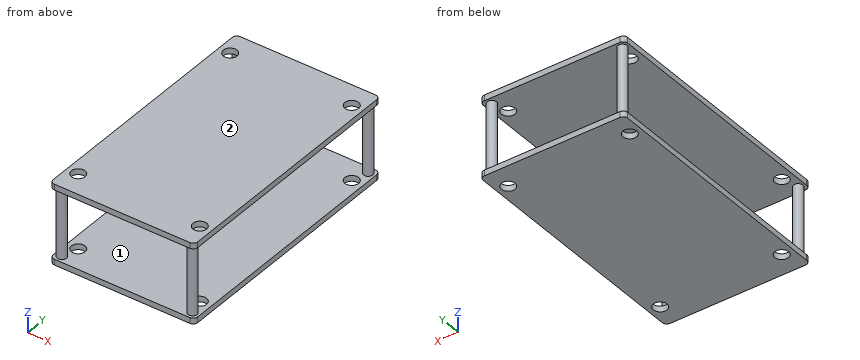
```python
from build123d import *

# Parameters (mm, degrees)
SKETCH1_W           = 63
SKETCH1_H           = 110
SKETCH1_R           = 3
BOSS_EXTRUDE1_DEPTH = 2.5
SKETCH3_R           = 2
BOSS_EXTRUDE3_DEPTH = 30
FILLET2_R           = 2
FILLET3_R           = 2
FILLET4_R           = 2
FILLET5_R           = 2
SKETCH5_W           = 63
SKETCH5_H           = 110
SKETCH5_R           = 3
BOSS_EXTRUDE5_DEPTH = 2.5
FILLET10_R          = 2
FILLET11_R          = 2
FILLET12_R          = 2
FILLET13_R          = 2


with BuildPart() as part:
    # Sketch1 → Boss-Extrude1 (new body)
    with BuildSketch(Plane.XY):
        Rectangle(SKETCH1_W, SKETCH1_H)
        with Locations((-26.5, 45)):
            Circle(SKETCH1_R, mode=Mode.SUBTRACT)
        with Locations((-26.5, -45)):
            Circle(SKETCH1_R, mode=Mode.SUBTRACT)
        with Locations((26.5, -45)):
            Circle(SKETCH1_R, mode=Mode.SUBTRACT)
        with Locations((26.5, 45)):
            Circle(SKETCH1_R, mode=Mode.SUBTRACT)
    extrude(amount=BOSS_EXTRUDE1_DEPTH)

    # Sketch3 → Boss-Extrude3 (add)
    with BuildSketch(Plane.XY.offset(2.5)):
        with Locations(Location((-28.5, 52, 0), (0, 0, 180))):
            Circle(SKETCH3_R)
        with Locations(Location((28.5, 52, 0), (0, 0, 180))):
            Circle(SKETCH3_R)
        with Locations(Location((28.5, -52, 0), (0, 0, 180))):
            Circle(SKETCH3_R)
        with Locations(Location((-28.5, -52, 0), (0, 0, 180))):
            Circle(SKETCH3_R)
    extrude(amount=BOSS_EXTRUDE3_DEPTH)

    # Fillet2
    fillet2_edges = [part.edges().sort_by_distance(p)[0] for p in [
        (31.5, -55, 1.25),
    ]]
    fillet(fillet2_edges, radius=FILLET2_R)

    # Fillet3
    fillet3_edges = [part.edges().sort_by_distance(p)[0] for p in [
        (31.5, 55, 1.25),
    ]]
    fillet(fillet3_edges, radius=FILLET3_R)

    # Fillet4
    fillet4_edges = [part.edges().sort_by_distance(p)[0] for p in [
        (-31.5, 55, 1.25),
    ]]
    fillet(fillet4_edges, radius=FILLET4_R)

    # Fillet5
    fillet5_edges = [part.edges().sort_by_distance(p)[0] for p in [
        (-31.5, -55, 1.25),
    ]]
    fillet(fillet5_edges, radius=FILLET5_R)

    # Sketch5 → Boss-Extrude5 (add)
    with BuildSketch(Plane.XY.offset(32.5)):
        Rectangle(SKETCH5_W, SKETCH5_H)
        with Locations((-26.5, 45)):
            Circle(SKETCH5_R, mode=Mode.SUBTRACT)
        with Locations((-26.5, -45)):
            Circle(SKETCH5_R, mode=Mode.SUBTRACT)
        with Locations((26.5, -45)):
            Circle(SKETCH5_R, mode=Mode.SUBTRACT)
        with Locations((26.5, 45)):
            Circle(SKETCH5_R, mode=Mode.SUBTRACT)
    extrude(amount=BOSS_EXTRUDE5_DEPTH)

    # Fillet10
    fillet10_edges = [part.edges().sort_by_distance(p)[0] for p in [
        (31.5, 55, 33.75),
    ]]
    fillet(fillet10_edges, radius=FILLET10_R)

    # Fillet11
    fillet11_edges = [part.edges().sort_by_distance(p)[0] for p in [
        (31.5, -55, 33.75),
    ]]
    fillet(fillet11_edges, radius=FILLET11_R)

    # Fillet12
    fillet12_edges = [part.edges().sort_by_distance(p)[0] for p in [
        (-31.5, -55, 33.75),
    ]]
    fillet(fillet12_edges, radius=FILLET12_R)

    # Fillet13
    fillet13_edges = [part.edges().sort_by_distance(p)[0] for p in [
        (-31.5, 55, 33.75),
    ]]
    fillet(fillet13_edges, radius=FILLET13_R)


solid = part.part
```
Verification items for the finished model (mm, model axes). Face numbers are marked on the shaded views. Coordinates: 2 decimals unless noted, no trailing zeros. Write each loop counter-clockwise with the first axis right and the second up, starting at its lowest first coordinate (ties: lowest second). Pieces come first, ordered by that corner, then holes. Notation, with made-up numbers: M 72.5,45 L 104.5,45 A9 cw 104.5,59 Z; hole C 38.25,88.25 d2. An arc over 180 degrees is marked long. Answer as a JSON object with one key per item and string values. Group by question number.
(1) Cross-section at D-D, the plane y = 22.5. Record the cut outline in (x, z), and give its area (3 significant figures).
(2) Cross-section at B-B, the plane x = -12. Record the cut outline in (y, z), and give its area (3 significant figures).
(3) Cross-section at A-A, the plane y = -45. Record the cut outline in (x, z), and give its area (3 significant figures).
(4) Material ranges on line 1 (Y direction, x = -26.5, z = 33.5); line 2 (Z direction, x = 20, y = 38), recorded low to high.
(5) Release check for a two-part mould opening along Y. For the marked faces 1 and 2 record: +Y half, -Y half, draft (parallel to the pull), parting line (faces both ways), or undercut.
(6) Cross-section at C-C, the plane z = 25. Record the cut outline in (x, y).
(7) Gauge pin test, flat end, axial feed: pin 1 (3.5 mm diameter, centred on x = -26.5, y = -45, fed in from +Z). Record the tip position at first contact, or that the pin passes through.
Reply:
{
 "1": {"outline": "M -31.5,0 L 31.5,0 L 31.5,2.5 L -31.5,2.5 Z; M -31.5,32.5 L 31.5,32.5 L 31.5,35 L -31.5,35 Z", "area": "315 mm²"},
 "2": {"outline": "M -55,0 L 55,0 L 55,2.5 L -55,2.5 Z; M -55,32.5 L 55,32.5 L 55,35 L -55,35 Z", "area": "550 mm²"},
 "3": {"outline": "M -31.5,0 L -29.5,0 L -29.5,2.5 L -31.5,2.5 Z; M -31.5,32.5 L -29.5,32.5 L -29.5,35 L -31.5,35 Z; M -23.5,0 L 23.5,0 L 23.5,2.5 L -23.5,2.5 Z; M -23.5,32.5 L 23.5,32.5 L 23.5,35 L -23.5,35 Z; M 29.5,0 L 31.5,0 L 31.5,2.5 L 29.5,2.5 Z; M 29.5,32.5 L 31.5,32.5 L 31.5,35 L 29.5,35 Z", "area": "255 mm²"},
 "4": {"line 1": "-55 to -48, -42 to 42, 48 to 55", "line 2": "0 to 2.5, 32.5 to 35"},
 "5": {"face 1": "undercut", "face 2": "draft"},
 "6": {"outline": "C -28.5,-52 d4; C -28.5,52 d4; C 28.5,-52 d4; C 28.5,52 d4"},
 "7": {"pin 1": "through"}
}
